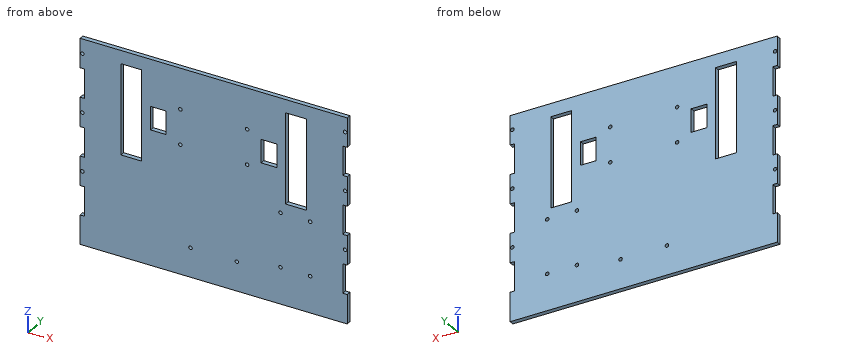
```python
from build123d import *

# Parameters (mm, degrees)
SKETCH1_R           = 1.524
SKETCH1_W           = 13.335
SKETCH1_H           = 20.32
SKETCH1_W_2         = 17.78
SKETCH1_H_2         = 78.74
BOSS_EXTRUDE1_DEPTH = 3.81


with BuildPart() as part:
    # Sketch1 → Boss-Extrude1 (new body)
    with BuildSketch(Plane(origin=(0, 0, 0), x_dir=(1, 0, 0), z_dir=(0, 1, 0))):
        Polygon((-114.3, -88.9), (114.3, -88.9), (114.3, -63.5), (110.49, -63.5), (110.49, -38.1), (114.3, -38.1), (114.3, -12.7), (110.49, -12.7), (110.49, 12.7), (114.3, 12.7), (114.3, 38.1), (110.49, 38.1), (110.49, 63.5), (114.3, 63.5), (114.3, 88.9), (-114.3, 88.9), (-114.3, 63.5), (-110.49, 63.5), (-110.49, 38.1), (-114.3, 38.1), (-114.3, 12.7), (-110.49, 12.7), (-110.49, -12.7), (-114.3, -12.7), (-114.3, -38.1), (-110.49, -38.1), (-110.49, -63.5), (-114.3, -63.5), align=None)
        with Locations((-28.575, -22.86)):
            Circle(SKETCH1_R, mode=Mode.SUBTRACT)
        with Locations((-28.575, -53.34)):
            Circle(SKETCH1_R, mode=Mode.SUBTRACT)
        with Locations((28.575, -53.34)):
            Circle(SKETCH1_R, mode=Mode.SUBTRACT)
        with Locations((28.575, -22.86)):
            Circle(SKETCH1_R, mode=Mode.SUBTRACT)
        with Locations((57.15, 57.15)):
            Circle(SKETCH1_R, mode=Mode.SUBTRACT)
        with Locations((57.15, 10.16)):
            Circle(SKETCH1_R, mode=Mode.SUBTRACT)
        with Locations((82.55, 10.16)):
            Circle(SKETCH1_R, mode=Mode.SUBTRACT)
        with Locations((82.55, 57.15)):
            Circle(SKETCH1_R, mode=Mode.SUBTRACT)
        with Locations((112.395, -76.2)):
            Circle(SKETCH1_R, mode=Mode.SUBTRACT)
        with Locations((-112.395, -76.2)):
            Circle(SKETCH1_R, mode=Mode.SUBTRACT)
        with Locations((-112.395, -25.4)):
            Circle(SKETCH1_R, mode=Mode.SUBTRACT)
        with Locations((-112.395, 25.4)):
            Circle(SKETCH1_R, mode=Mode.SUBTRACT)
        with Locations((112.395, -25.4)):
            Circle(SKETCH1_R, mode=Mode.SUBTRACT)
        with Locations((112.395, 25.4)):
            Circle(SKETCH1_R, mode=Mode.SUBTRACT)
        with Locations((-19.8501, 63.5)):
            Circle(SKETCH1_R, mode=Mode.SUBTRACT)
        with Locations((19.8501, 63.5)):
            Circle(SKETCH1_R, mode=Mode.SUBTRACT)
        with Locations((-47.3075, -38.1)):
            Rectangle(SKETCH1_W, SKETCH1_H, mode=Mode.SUBTRACT)
        with Locations((70.485, -38.1)):
            Rectangle(SKETCH1_W_2, SKETCH1_H_2, mode=Mode.SUBTRACT)
        with Locations((-70.485, -38.1)):
            Rectangle(SKETCH1_W_2, SKETCH1_H_2, mode=Mode.SUBTRACT)
        with Locations((47.3075, -38.1)):
            Rectangle(SKETCH1_W, SKETCH1_H, mode=Mode.SUBTRACT)
    extrude(amount=BOSS_EXTRUDE1_DEPTH)


solid = part.part
```
Check sheet for the modelled part. Datum: model origin and axes. Units: mm. Round coordinates to 2 decimals unless told otherwise and drop trailing zeros. Order: outer loops, then holes, each group sorted by start corner. A loop starts at its lowest first (then second) coordinate and runs counter-clockwise, first axis right, second up. Notation, with made-up numbers: (0, 65) -> (49, 65) arc R22 ccw to (49, 71) -> close; hole circle Ø1 at (13, 87). An arc over 180 degrees is marked (long way). One line per item, written item: value. Start each with the question number.
Q1. Cross-section at B-B (y = 3.15). Give the number of separate pieces and of enclosed holes in the cut face, and give its area (3 significant figures).
Q2. Thickness scan on line 1 (X direction, y = 3.3, z = 19.5) (3 decimals); line 2 (X direction, y = 1.6, z = 63) (3 decimals); line 3 (X direction, y = 2.3, z = 53.34) (3 decimals). Record the ranges inside material, lowest first.
Q3. Cross-section at A-A (x = 76). Record the boundary of the cut face in (y, z), and give its area (3 significant figures).
Q4. Gauge pin test, flat end, axial feed: pin 1 Ø1.9 at (y, z) = (2, 47) entering from +X. Record the tip position at first contact, or that the pin passes through.
Completed:
1. separate pieces: 1
1. enclosed holes: 20
1. area: 36,600 mm²
2. line 1: x = -114.3 to -79.375, -61.595 to 61.595, 79.375 to 114.3
2. line 2: x = -110.49 to -79.375, -61.595 to 61.595, 79.375 to 110.49
2. line 3: x = -110.49 to -79.375, -61.595 to -30.099, -27.051 to 27.051, 30.099 to 61.595, 79.375 to 110.49
3. outline: (0, -88.9) -> (3.81, -88.9) -> (3.81, -1.27) -> (0, -1.27) -> close; (0, 77.47) -> (3.81, 77.47) -> (3.81, 88.9) -> (0, 88.9) -> close
3. area: 377 mm²
4. pin 1: stops at x = 110.49
